```python
from build123d import *

# Parameters (mm, degrees)
F0_R     = 6.35
F1_DEPTH = 873.125
F2_W     = 6.6555930256
F2_H     = 6.604
F3_DEPTH = 12.7


with BuildPart() as f1:
    # F0 (on Front) → F1 (new body, symmetric)
    with BuildSketch(Plane.XZ):
        Circle(F0_R)
    extrude(amount=F1_DEPTH, both=True)

    # F2 (on Right) → F3 (cut, symmetric)
    with BuildSketch(Plane.YZ):
        with Locations((-872.6427965128, 0)):
            Rectangle(F2_W, F2_H)
    extrude(amount=F3_DEPTH, both=True, mode=Mode.SUBTRACT)


solid = f1.part
```
The model under review builds one solid part; all positions refer to its coordinate system, in mm. Give positions to 0.01 mm unless a question says otherwise; leave off trailing zeros. Write each loop counter-clockwise with the first axis right and the second up, starting at its lowest first coordinate (ties: lowest second). Pieces come first, ordered by that corner, then holes. Notation, with made-up numbers: (17, -18.5) - (24, -18.5) arc R20 cw to (24, -1.5) - close; hole circle Ø7 at (-0.5, 14.25). An arc over 180 degrees is marked (long way). Answer in a Markdown table with one row per item. Add a question column.
1. Wall thickness on line 1 along Z through (x, y) = (5.5, 140.5); line 2 along Z through (x, y) = (-2, 613); line 3 along X through (y, z) = (-431.5, -0.25): over which ranges is each line inside the solid? List them lowest first. Write a range as [from, to].
2. We need section A-A on x = 3. Write out the cut boundary in (y, z) (3 decimals).
3. Insertion check: P1, Ø1.5, axis at x = 5, y = 126.5, coming from the +Z side; P2, Ø3, axis at x = -3, y = 466, coming from the +Z side; P3, Ø3.5, axis at x = -2, z = 0, coming from the -Y side (3 decimals). Each pin has a flat end and moves straight along its axis. Give the tip position at first contact, or say it passes through.
4. We need section B-B on y = -366.5. Write out the cut boundary in (x, z), then the cut area to 3 significant figures.
Ans:
| question | item | result |
|---|---|---|
| 1 | line 1 | z = [-3.17, 3.17] |
| 1 | line 2 | z = [-6.03, 6.03] |
| 1 | line 3 | x = [-6.35, 6.35] |
| 2 | outline | (-873.125, -5.597) - (873.125, -5.597) - (873.125, 5.597) - (-873.125, 5.597) - (-873.125, 3.302) - (-869.315, 3.302) - (-869.315, -3.302) - (-873.125, -3.302) - close |
| 3 | P1 | stops at z = 4.72 |
| 3 | P2 | stops at z = 6.17 |
| 3 | P3 | stops at y = -869.315 |
| 4 | outline | circle Ø12.7 at (0, 0) |
| 4 | area | 127 mm^2 |
